Geometry: see drawing. Coordinates: mm, zero at the bounding-box minimum. Give positions to 0.01 mm unless a question says otherwise; leave off trailing zeros. Loops run counter-clockwise (first coordinate to the right, second up) from the corner with the lowest first, then second, coordinate; pieces in that order, holes last. Notation, with made-up numbers: (-24.75, 1.25) - (2.25, 1.25) arc R18 cw to (2.25, 13.25) - close; hole circle Ø2 at (64, -5.75). An arc over 180 degrees is marked (long way). Use CSV: the item, a comma, the result in double quotes. Start each with the question number.
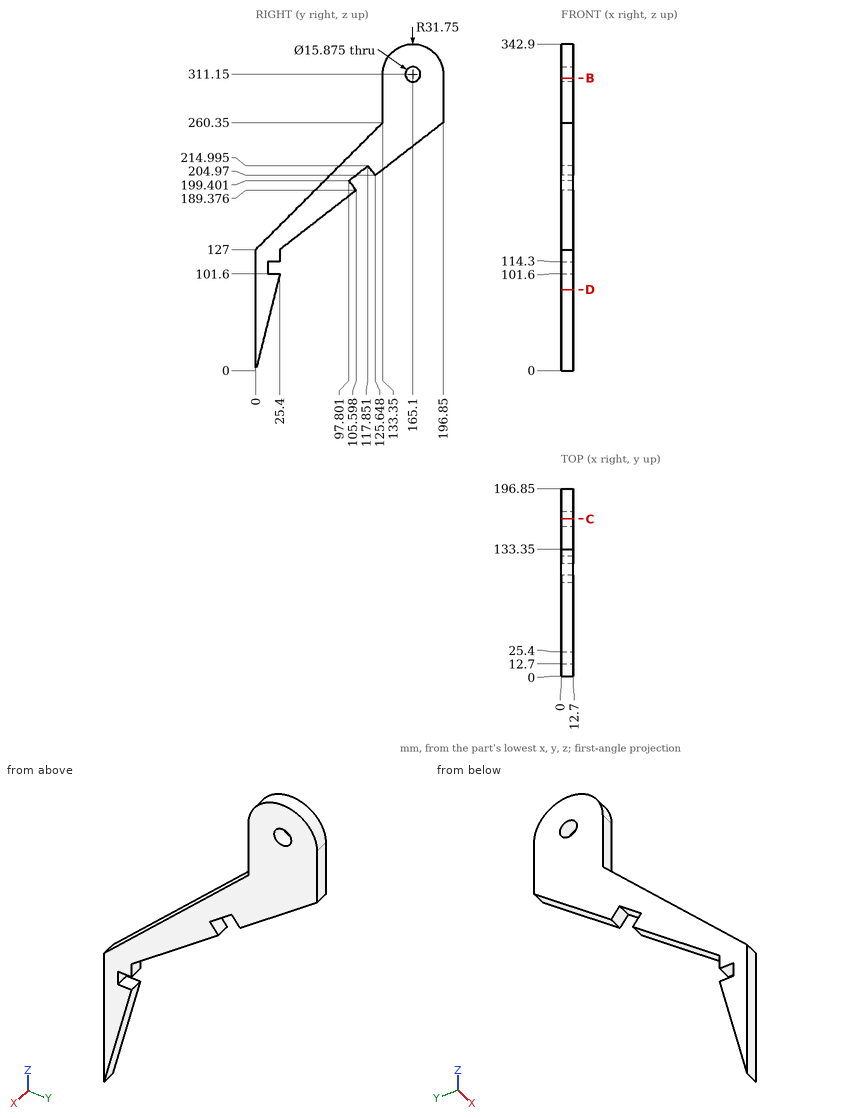
Item 1: Pin query (flat end, axial travel): pin 1 Ø1 at (x, z) = (10.5, 165) entering from +Y; pin 2 Ø6.5 at (x, z) = (7.5, 110.5) entering from +Y; pin 3 Ø6 at (x, y) = (10, 159) entering from -Z. Return the tip coordinate at first contact, or that it passes through.
Item 2: Section D-D (z = 85). Output: boundary loops of the cut face in (x, y), plus the area to 3 significant figures.
Item 3: Section C-C (y = 165.1). Output: boundary loops of the cut face in (x, z) (1 decimal), plus the area to 3 significant figures.
Item 4: Ray query, probe 1 along Y at (x, z) = (2.5, 311.15); probe 2 along Y at (x, z) = (1.5, 126); probe 3 along Y at (x, z) = (12, 32). Return the intervals inside material, ascending.
Item 5: Section B-B (z = 307). Output: boundary loops of the cut face in (x, y).
Outcome:
1,pin 1,"stops at y = 74.9"
1,pin 2,"stops at y = 12.7"
1,pin 3,"stops at z = 228.58"
2,outline,"(0, 0) - (12.7, 0) - (12.7, 21.25) - (0, 21.25) - close"
2,area,"270 mm2"
3,outline,"(0, 235.7) - (12.7, 235.7) - (12.7, 303.2) - (0, 303.2) - close; (0, 319.1) - (12.7, 319.1) - (12.7, 342.9) - (0, 342.9) - close"
3,area,"1,160 mm2"
4,probe 1,"y = 133.35 to 157.16, 173.04 to 196.85"
4,probe 2,"y = 0 to 25.4"
4,probe 3,"y = 0 to 8"
5,outline,"(0, 133.35) - (12.7, 133.35) - (12.7, 158.33) - (0, 158.33) - close; (0, 171.87) - (12.7, 171.87) - (12.7, 196.85) - (0, 196.85) - close"
